from build123d import *

# Parameters (mm, degrees)
SKETCH1_W           = 52.300000048
SKETCH1_H           = 139.7
BOSS_EXTRUDE1_DEPTH = 3.175
BOSS_EXTRUDE2_DEPTH = 52.300000048


with BuildPart() as part:
    # Sketch1 → Boss-Extrude1 (new body)
    with BuildSketch(Plane(origin=(0, 0, 0), x_dir=(0, 0, -1), z_dir=(1, 0, 0))):
        with Locations((26.150000024, 69.85)):
            Rectangle(SKETCH1_W, SKETCH1_H)
    extrude(amount=BOSS_EXTRUDE1_DEPTH)

    # Sketch2 → Boss-Extrude2 (add)
    with BuildSketch(Plane(origin=(0, 0, -52.300000048), x_dir=(-1, 0, 0), z_dir=(0, 0, -1))):
        with BuildLine():
            Line((9.525, -9.525), (9.525, -12.7))
            ThreePointArc((9.525, -12.7), (0.544743879, -8.980256121), (-3.175, 0))
            Line((-3.175, 0), (0, 0))
            ThreePointArc((0, 0), (2.789807909, -6.735192091), (9.525, -9.525))
        make_face()
        with BuildLine():
            Line((0, 139.7), (-3.175, 139.7))
            ThreePointArc((-3.175, 139.7), (0.544743879, 148.680256121), (9.525, 152.4))
            Line((9.525, 152.4), (9.525, 149.225))
            ThreePointArc((9.525, 149.225), (2.789807909, 146.435192091), (0, 139.7))
        make_face()
    extrude(amount=-BOSS_EXTRUDE2_DEPTH)


solid = part.part
The model under review builds one solid part; all positions refer to its coordinate system, in mm. A direction names the side the tool comes from. Coordinates: 2 decimals unless noted, no trailing zeros. Loops run counter-clockwise (first coordinate to the right, second up) from the corner with the lowest first, then second, coordinate; pieces in that order, holes last.
(1) Insertion check: P1, Ø6, axis at x = -0.5, z = -21.5, coming from the -Y side; P2, Ø2, axis at x = 0, z = -5, coming from the +Y side; P3, Ø12, axis at y = 52.5, z = -40, coming from the -X side. Each pin has a flat end and moves straight along its axis. Give the tip position at first contact, or say it passes through.
Determined:
P1: stops at y = -11.18
P2: stops at y = 149.11
P3: stops at x = 0
(2) Consider section C-C, the plane y = 107. Give the boundary of the cut face in (x, z) (3 decimals).
Determined:
outline: (0, -52.3) - (3.175, -52.3) - (3.175, 0) - (0, 0) - close
(3) Wall thickness on L1, parallel to X at y = 32.5, z = -28 (3 decimals); L2, parallel to Y at x = -4.75, z = -17.5; L3, parallel to Y at x = -8.5, z = -10.5: over which ranges is each line inside the solid? List them lowest first.
Determined:
L1: x = 0 to 3.175
L2: y = -11.77 to -8.24, 147.94 to 151.47
L3: y = -12.66 to -9.47, 149.17 to 152.36
(4) Consider section A-A, the plane z = -13.5. Give the boundary of the cut face in (x, y) (3 decimals).
Determined:
outline: (-9.525, -12.7) arc R12.7 ccw to (3.175, 0) - (3.175, 139.7) arc R12.7 ccw to (-9.525, 152.4) - (-9.525, 149.225) arc R9.525 cw to (0, 139.7) - (0, 0) arc R9.525 cw to (-9.525, -9.525) - close
(5) Draft analysis for pull direction Y (two halves, no side actions). For faces 3 (the cylindrical face through (-0.644, -9.078, -26.516)), 4 (the flat face through (0, 71, -26)), 5 (the cylindrical face through (-2.864, 146.509, -26.516)), 6 (the flat face through (2, 70, -52.3)), state which applies: +Y half, -Y half, draft (parallel to the pull), parting line (faces both ways), or undercut.
Determined:
face 3: -Y half
face 4: undercut
face 5: undercut
face 6: draft
(6) Tool access review of faces 1 (the cylindrical face through (-2.716, -6.661, -26.516)), 2 (the cylindrical face through (-0.447, 148.581, -26.516)): name each direction out of +Z, -Z, +X, -X, +Y, -Y from which nothing blocks a thin tool from reaching the whole face with its end or side.
Determined:
face 1: +Z, -Z, -X
face 2: +Z, -Z, +X, +Y
(7) Consider section B-B, the plane x = -6.5. Give the boundary of the cut face in (y, z), plus the area to 3 significant figures.
Determined:
outline: (-12.33, -52.3) - (-9.03, -52.3) - (-9.03, 0) - (-12.33, 0) - close; (148.73, -52.3) - (152.03, -52.3) - (152.03, 0) - (148.73, 0) - close
area: 345 mm2
